from build123d import *

# Parameters (mm, degrees)
SKETCH1_R                    = 6.35
BOSS_EXTRUDE1_DEPTH          = 6.35
F_1_8_0_125_DIAMETER_HOLE1_D = 3.175
SKETCH4_R                    = 1.5875
BOSS_EXTRUDE2_DEPTH          = 4.7625


with BuildPart() as part:
    # Sketch1 → Boss-Extrude1 (new body)
    with BuildSketch(Plane(origin=(0, 0, 0), x_dir=(1, 0, 0), z_dir=(0, 1, 0))):
        with Locations(Location((0, 0, 0), (0, 0, 270))):
            Circle(SKETCH1_R)
    extrude(amount=BOSS_EXTRUDE1_DEPTH)

    # 1/8 (0.125) Diameter Hole1 (through all)
    with Locations(Plane(origin=(0, 6.35, 0), x_dir=(1, 0, 0), z_dir=(0, 1, 0))):
        with Locations((0, 0)):
            Hole(F_1_8_0_125_DIAMETER_HOLE1_D / 2)

    # Sketch4 → Boss-Extrude2 (add)
    with BuildSketch(Plane(origin=(0, 6.35, 0), x_dir=(1, 0, 0), z_dir=(0, 1, 0))):
        with Locations(Location((3.96875, 0, 0), (0, 0, 90))):
            Circle(SKETCH4_R)
        with Locations(Location((-3.96875, 0, 0), (0, 0, 90))):
            Circle(SKETCH4_R)
    extrude(amount=BOSS_EXTRUDE2_DEPTH)


solid = part.part
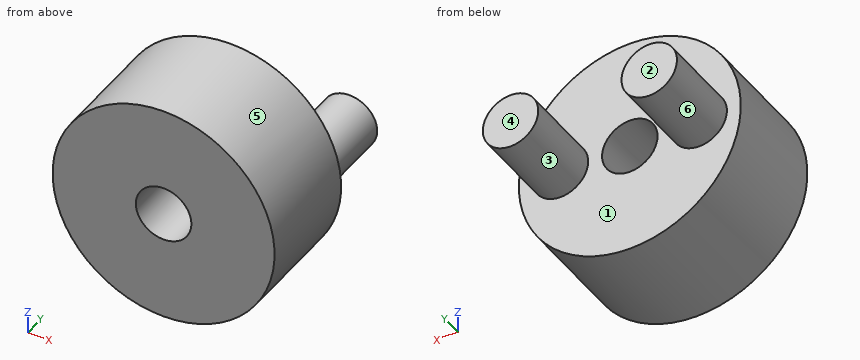
Could you check a few things on this model? Use its own coordinates, in mm. Face numbers are marked on the shaded views. A direction names the side the tool comes from. Give positions to 0.01 mm unless a question says otherwise; leave off trailing zeros. Order: outer loops, then holes, each group sorted by start corner. A loop starts at its lowest first (then second) coordinate and runs counter-clockwise, first axis right, second up.
1. Suppose I cut it at D-D (x = 3). Write out the boundary of the cut face in (y, z).
Answers below:
outline: (0, -5.6) - (6.35, -5.6) - (6.35, -1.26) - (11.11, -1.26) - (11.11, 1.26) - (6.35, 1.26) - (6.35, 5.6) - (0, 5.6) - close
2. Suppose I cut it at B-B (x = -3.5). Write out the boundary of the cut face in (y, z), plus the area to 3 significant figures.
Answers below:
outline: (0, -5.3) - (6.35, -5.3) - (6.35, -1.52) - (11.11, -1.52) - (11.11, 1.52) - (6.35, 1.52) - (6.35, 5.3) - (0, 5.3) - close
area: 81.7 mm2
3. I need wall thicknesses on L1, parallel to X at y = 7.25, z = 0; L2, parallel to Y at x = -3.75, z = 2; L3, parallel to X at y = 10, z = -1. Which ranges of each line are inside material? Lowest first, please.
Answers below:
L1: x = -5.56 to -2.38, 2.38 to 5.56
L2: y = 0 to 6.35
L3: x = -5.2 to -2.74, 2.74 to 5.2
4. Which directions (+Z, -Z, +X, -X, +Y, -Y) give clear straight access to the entire face, cutting with the end or side of a thin tool? Please do the marked faces 1 and 2.
Answers below:
face 1: +Y
face 2: +Z, -Z, +X, -X, +Y
5. For pin 1 (5 mm diameter, centred on x = -3, y = 7, fed in from -Z); pin 2 (2 mm diameter, centred on y = 7, z = -4, fed in from -X); pin 3 (3 mm diameter, centred on x = 0, z = 0, fed in from +Y); pin 4 (1.5 mm diameter, centred on x = -3, y = 9, fed in from +Z), each with a flat end and sliding along its axis, tell me the tip position at first contact or that it passes through.
Answers below:
pin 1: stops at z = -6.32
pin 2: stops at x = -5.46
pin 3: passes through
pin 4: stops at z = 1.57
6. Thinking about a two-plate mould opening in X: for the marked faces 3, 4, 5 and 6, which applies, +X half, -X half, draft (parallel to the pull), parting line (faces both ways), or undercut?
Answers below:
face 3: undercut
face 4: draft
face 5: parting line
face 6: undercut
7. Suppose I cut it at A-A (z = 0). Write out the boundary of the cut face in (x, y).
Answers below:
outline: (-6.35, 0) - (-1.59, 0) - (-1.59, 6.35) - (-2.38, 6.35) - (-2.38, 11.11) - (-5.56, 11.11) - (-5.56, 6.35) - (-6.35, 6.35) - close; (1.59, 0) - (6.35, 0) - (6.35, 6.35) - (5.56, 6.35) - (5.56, 11.11) - (2.38, 11.11) - (2.38, 6.35) - (1.59, 6.35) - close
